```python
from build123d import *

# Parameters (mm, degrees)
F0_W     = 901.7
F0_H     = 298.45
F1_DEPTH = 3.175
F2_R     = 8.001
F3_DEPTH = 6.351


with BuildPart() as f1:
    # F0 (on Front) → F1 (new body, symmetric)
    with BuildSketch(Plane.XZ):
        Rectangle(F0_W, F0_H)
    extrude(amount=F1_DEPTH, both=True)

    # F2 (on face) → F3 (cut, through all)
    with BuildSketch(Plane.XZ.offset(3.175)):
        with Locations((-431.8, -123.825)):
            Circle(F2_R)
        with Locations((-431.8, -73.025)):
            Circle(F2_R)
        with Locations((-431.8, -22.225)):
            Circle(F2_R)
        with Locations((-431.8, 28.575)):
            Circle(F2_R)
        with Locations((-431.8, 79.375)):
            Circle(F2_R)
        with Locations((-431.8, 130.175)):
            Circle(F2_R)
        with Locations((-381, -123.825)):
            Circle(F2_R)
        with Locations((-381, -73.025)):
            Circle(F2_R)
        with Locations((-381, -22.225)):
            Circle(F2_R)
        with Locations((-381, 28.575)):
            Circle(F2_R)
        with Locations((-381, 79.375)):
            Circle(F2_R)
        with Locations((-381, 130.175)):
            Circle(F2_R)
        with Locations((-330.2, -123.825)):
            Circle(F2_R)
        with Locations((-330.2, -73.025)):
            Circle(F2_R)
        with Locations((-330.2, -22.225)):
            Circle(F2_R)
        with Locations((-330.2, 28.575)):
            Circle(F2_R)
        with Locations((-330.2, 79.375)):
            Circle(F2_R)
        with Locations((-330.2, 130.175)):
            Circle(F2_R)
        with Locations((-279.4, -123.825)):
            Circle(F2_R)
        with Locations((-279.4, -73.025)):
            Circle(F2_R)
        with Locations((-279.4, -22.225)):
            Circle(F2_R)
        with Locations((-279.4, 28.575)):
            Circle(F2_R)
        with Locations((-279.4, 79.375)):
            Circle(F2_R)
        with Locations((-279.4, 130.175)):
            Circle(F2_R)
        with Locations((-228.6, -123.825)):
            Circle(F2_R)
        with Locations((-228.6, -73.025)):
            Circle(F2_R)
        with Locations((-228.6, -22.225)):
            Circle(F2_R)
        with Locations((-228.6, 28.575)):
            Circle(F2_R)
        with Locations((-228.6, 79.375)):
            Circle(F2_R)
        with Locations((-228.6, 130.175)):
            Circle(F2_R)
        with Locations((-177.8, -123.825)):
            Circle(F2_R)
        with Locations((-177.8, -73.025)):
            Circle(F2_R)
        with Locations((-177.8, -22.225)):
            Circle(F2_R)
        with Locations((-177.8, 28.575)):
            Circle(F2_R)
        with Locations((-177.8, 79.375)):
            Circle(F2_R)
        with Locations((-177.8, 130.175)):
            Circle(F2_R)
        with Locations((-127, -123.825)):
            Circle(F2_R)
        with Locations((-127, -73.025)):
            Circle(F2_R)
        with Locations((-127, -22.225)):
            Circle(F2_R)
        with Locations((-127, 28.575)):
            Circle(F2_R)
        with Locations((-127, 79.375)):
            Circle(F2_R)
        with Locations((-127, 130.175)):
            Circle(F2_R)
        with Locations((-76.2, -123.825)):
            Circle(F2_R)
        with Locations((-76.2, -73.025)):
            Circle(F2_R)
        with Locations((-76.2, -22.225)):
            Circle(F2_R)
        with Locations((-76.2, 28.575)):
            Circle(F2_R)
        with Locations((-76.2, 79.375)):
            Circle(F2_R)
        with Locations((-76.2, 130.175)):
            Circle(F2_R)
        with Locations((-25.4, -123.825)):
            Circle(F2_R)
        with Locations((-25.4, -73.025)):
            Circle(F2_R)
        with Locations((-25.4, -22.225)):
            Circle(F2_R)
        with Locations((-25.4, 28.575)):
            Circle(F2_R)
        with Locations((-25.4, 79.375)):
            Circle(F2_R)
        with Locations((-25.4, 130.175)):
            Circle(F2_R)
        with Locations((25.4, -123.825)):
            Circle(F2_R)
        with Locations((25.4, -73.025)):
            Circle(F2_R)
        with Locations((25.4, -22.225)):
            Circle(F2_R)
        with Locations((25.4, 28.575)):
            Circle(F2_R)
        with Locations((25.4, 79.375)):
            Circle(F2_R)
        with Locations((25.4, 130.175)):
            Circle(F2_R)
        with Locations((76.2, -123.825)):
            Circle(F2_R)
        with Locations((76.2, -73.025)):
            Circle(F2_R)
        with Locations((76.2, -22.225)):
            Circle(F2_R)
        with Locations((76.2, 28.575)):
            Circle(F2_R)
        with Locations((76.2, 79.375)):
            Circle(F2_R)
        with Locations((76.2, 130.175)):
            Circle(F2_R)
        with Locations((127, -123.825)):
            Circle(F2_R)
        with Locations((127, -73.025)):
            Circle(F2_R)
        with Locations((127, -22.225)):
            Circle(F2_R)
        with Locations((127, 28.575)):
            Circle(F2_R)
        with Locations((127, 79.375)):
            Circle(F2_R)
        with Locations((127, 130.175)):
            Circle(F2_R)
        with Locations((177.8, -123.825)):
            Circle(F2_R)
        with Locations((177.8, -73.025)):
            Circle(F2_R)
        with Locations((177.8, -22.225)):
            Circle(F2_R)
        with Locations((177.8, 28.575)):
            Circle(F2_R)
        with Locations((177.8, 79.375)):
            Circle(F2_R)
        with Locations((177.8, 130.175)):
            Circle(F2_R)
        with Locations((228.6, -123.825)):
            Circle(F2_R)
        with Locations((228.6, -73.025)):
            Circle(F2_R)
        with Locations((228.6, -22.225)):
            Circle(F2_R)
        with Locations((228.6, 28.575)):
            Circle(F2_R)
        with Locations((228.6, 79.375)):
            Circle(F2_R)
        with Locations((228.6, 130.175)):
            Circle(F2_R)
        with Locations((279.4, -123.825)):
            Circle(F2_R)
        with Locations((279.4, -73.025)):
            Circle(F2_R)
        with Locations((279.4, -22.225)):
            Circle(F2_R)
        with Locations((279.4, 28.575)):
            Circle(F2_R)
        with Locations((279.4, 79.375)):
            Circle(F2_R)
        with Locations((279.4, 130.175)):
            Circle(F2_R)
        with Locations((330.2, -123.825)):
            Circle(F2_R)
        with Locations((330.2, -73.025)):
            Circle(F2_R)
        with Locations((330.2, -22.225)):
            Circle(F2_R)
        with Locations((330.2, 28.575)):
            Circle(F2_R)
        with Locations((330.2, 79.375)):
            Circle(F2_R)
        with Locations((330.2, 130.175)):
            Circle(F2_R)
        with Locations((381, -123.825)):
            Circle(F2_R)
        with Locations((381, -73.025)):
            Circle(F2_R)
        with Locations((381, -22.225)):
            Circle(F2_R)
        with Locations((381, 28.575)):
            Circle(F2_R)
        with Locations((381, 79.375)):
            Circle(F2_R)
        with Locations((381, 130.175)):
            Circle(F2_R)
        with Locations((431.8, -123.825)):
            Circle(F2_R)
        with Locations((431.8, -73.025)):
            Circle(F2_R)
        with Locations((431.8, -22.225)):
            Circle(F2_R)
        with Locations((431.8, 28.575)):
            Circle(F2_R)
        with Locations((431.8, 79.375)):
            Circle(F2_R)
        with Locations((431.8, 130.175)):
            Circle(F2_R)
    extrude(amount=-F3_DEPTH, mode=Mode.SUBTRACT)


solid = f1.part
```
The listing builds one solid part. Answer for the finished solid, in the listing's coordinates (mm). Coordinates: 2 decimals unless noted, no trailing zeros. Loops run counter-clockwise (first coordinate to the right, second up) from the corner with the lowest first, then second, coordinate; pieces in that order, holes last. Notation, with made-up numbers: (3.25, 16.25) - (53.25, 16.25) arc R28 cw to (53.25, 35.25) - close; hole circle Ø11 at (30, 71). An arc over 180 degrees is marked (long way). Use a Markdown table: item, result. Add a question column.
1) The part is cut by section B-B, the plane y = -0.25. State how many separate pieces and enclosed holes the cut face has, and give its area (3 significant figures).
2) The part is cut by section A-A, the plane x = -177.8. Give the vertices of the cut face in (y, z) (3 decimals), and give its area (3 significant figures).
3) The mould has two halves that part along X. Classify faces 1 (the flat face through (-6, 3.175, 2)), 2 (the cylindrical face through (83.59, -0.04, -25.29)): released by +X, released by -X, zero draft, split by the parting line, or undercut.
Here are the results:
| question | item | result |
|---|---|---|
| 1 | separate pieces | 1 |
| 1 | enclosed holes | 108 |
| 1 | area | 247,000 mm^2 |
| 2 | outline | (-3.175, -149.225) - (3.175, -149.225) - (3.175, -131.826) - (-3.175, -131.826) - close; (-3.175, -115.824) - (3.175, -115.824) - (3.175, -81.026) - (-3.175, -81.026) - close; (-3.175, -65.024) - (3.175, -65.024) - (3.175, -30.226) - (-3.175, -30.226) - close; (-3.175, -14.224) - (3.175, -14.224) - (3.175, 20.574) - (-3.175, 20.574) - close; (-3.175, 36.576) - (3.175, 36.576) - (3.175, 71.374) - (-3.175, 71.374) - close; (-3.175, 87.376) - (3.175, 87.376) - (3.175, 122.174) - (-3.175, 122.174) - close; (-3.175, 138.176) - (3.175, 138.176) - (3.175, 149.225) - (-3.175, 149.225) - close |
| 2 | area | 1,290 mm^2 |
| 3 | face 1 | zero draft |
| 3 | face 2 | undercut |
